Autodesk Fusion 360 part; units mm, degrees
sketch "Sketch1" plane through (0, 0, 0) normal (0, 0, 1) x (1, 0, 0)
  line L0 (-5.15, 5.15) -> (5.15, 5.15)
  line L1 (5.15, 5.15) -> (5.15, -5.15)
  line L2 (5.15, -5.15) -> (-5.15, -5.15)
  line L3 (-5.15, -5.15) -> (-5.15, 5.15)
  dimension "d1" = 10.3
  dimension "d2" = 10.3
  dimension "d3" = 5.15
  dimension "d4" = 5.15
extrude "Extrude1" add sketch "Sketch1" along normal blind 3.7
sketch "Sketch2" plane through (0, 0, 0) normal (0, 1, 0) x (1, 0, 0)
  line L0 (-5.15, -3.7) -> (5.15, -3.7)
  line L1 (0, -3.7) -> (0, -6.6)
  line L2 (5.15, 0) -> (-5.15, 0)
  line L3 (0, -3.7) -> (4.8, -3.7)
  arc A0 (0, -6.6) -> (4.8, -3.7) centre (-0.149, -0.931) ccw
  dimension "d7" = 6.6
  dimension "d8" = 4.8
revolve "Revolve1" add sketch "Sketch2" angle 360 about axis through (0, 0, 3.7) along (0, 0, 1)
fillet "Fillet1" radius 1 4 edges at (5.15, -5.15, 1.85) (5.15, 5.15, 1.85) (-5.15, 5.15, 1.85) (-5.15, -5.15, 1.85)
equation "d3 = d1 / 2"
equation "d4 = d2 / 2"
equation "d8 = ( 9.6 / 2 ) * 1 mm"
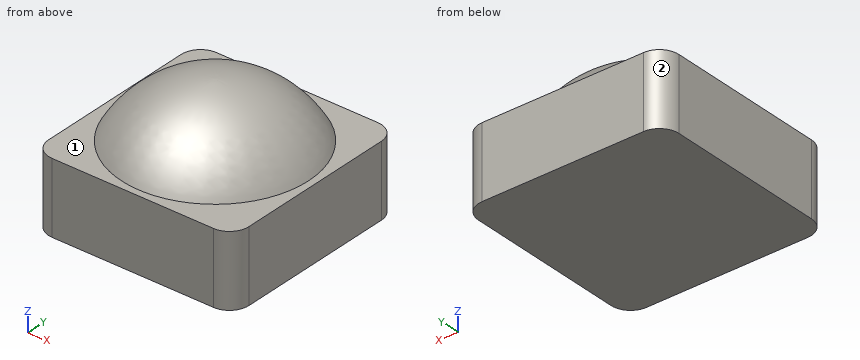
Verification items for the finished model (mm, model axes). Face numbers are marked on the shaded views. A direction names the side the tool comes from. Coordinates: 2 decimals unless noted, no trailing zeros. Return JSON: item names as keys, results as strings.
1. Thickness scan on L1, parallel to Z at x = 4, y = -2.75; L2, parallel to Z at x = -1.25, y = -2.5; L3, parallel to Y at x = -4, z = 3.75. Record the ranges inside material, lowest first.
Established:
{"L1": "z = 0 to 3.7", "L2": "z = 0 to 5.78", "L3": "y = -2.6 to 2.6"}
2. Tool access check on the marked faces 1 and 2. Record the directions out of +Z, -Z, +X, -X, +Y, -Y that give a thin tool (end or side, any length) a straight path to the whole face; none if there is none.
Established:
{"face 1": "+Z", "face 2": "+Z, -Z, -X, +Y"}
3. Go/stop test with flat-tipped pins: pin 1 (2 mm diameter, centred on x = 3, z = 6, fed in from -Y); pin 2 (5 mm diameter, centred on x = -2.5, y = 2.5, fed in from +Z). Record where each tip stops, or that it passes through.
Established:
{"pin 1": "stops at y = -2.67", "pin 2": "stops at z = 6.48"}
